The model under review builds one solid part; all positions refer to its coordinate system, in mm. A direction names the side the tool comes from. Coordinates: 2 decimals unless noted, no trailing zeros. Loops run counter-clockwise (first coordinate to the right, second up) from the corner with the lowest first, then second, coordinate; pieces in that order, holes last. Notation, with made-up numbers: M 26.25,17 L 42.25,17 A14 ccw 42.25,33 Z; hole C 71,86.5 d6. An arc over 180 degrees is marked long. Use one line per item in the form item = value.
```python
from build123d import *

# Parameters (mm, degrees)
F0_W     = 57
F0_H     = 44
F1_DEPTH = 167
F2_W     = 53
F2_H     = 40
F3_DEPTH = 165
F4_W     = 20
F4_H     = 15
F5_DEPTH = 84
F6_W     = 10
F6_H     = 80
F7_DEPTH = 2


with BuildPart() as f1:
    # F0 (on Top) → F1 (new body)
    with BuildSketch(Plane.XY):
        Rectangle(F0_W, F0_H)
    extrude(amount=F1_DEPTH)

    # F2 (on face) → F3 (cut)
    with BuildSketch(Plane.XY.offset(167)):
        Rectangle(F2_W, F2_H)
    extrude(amount=-F3_DEPTH, mode=Mode.SUBTRACT)

    # F4 (on face) → F5 (cut)
    with BuildSketch(Plane.YZ.offset(28.5)):
        with Locations((-12, 9.5)):
            Rectangle(F4_W, F4_H)
    extrude(amount=-F5_DEPTH, mode=Mode.SUBTRACT)

    # F6 (on face) → F7 (cut)
    with BuildSketch(Plane.XZ.offset(22)):
        Polygon((5, 49.017786), (-5, 49.017786), (0, 40.357532), align=None)
        with Locations((0, 89.017786)):
            Rectangle(F6_W, F6_H)
        Polygon((0, 137.67804), (-5, 129.017786), (5, 129.017786), align=None)
    extrude(amount=-F7_DEPTH, mode=Mode.SUBTRACT)


solid = f1.part
```
1. Add section B-B (z = 30). State the section outline as (x, y) points, then the cut area to 3 significant figures.
Response values:
outline = M -28.5,-22 L 28.5,-22 L 28.5,22 L -28.5,22 Z; hole M -26.5,-20 L 26.5,-20 L 26.5,20 L -26.5,20 Z
area = 388 mm^2
2. Wall thickness on line 1 along X through (y, z) = (11, 65); line 2 along Y through (x, z) = (-25.5, 136.5); line 3 along Z through (x, y) = (-18, -1): over which ranges is each line inside the solid? List them lowest first. Write a range as from..to.
Response values:
line_1 = -28.5..-26.5, 26.5..28.5
line_2 = -22..-20, 20..22
line_3 = 0..2
3. Add section A-A (x = -7). State the section outline as (y, z) points, then the cut area to 3 significant figures.
Response values:
outline = M -22,0 L 22,0 L 22,167 L 20,167 L 20,2 L -22,2 Z; M -22,17 L -20,17 L -20,167 L -22,167 Z
area = 718 mm^2
4. Add section D-D (x = 2). State the section outline as (y, z) points.
Response values:
outline = M -22,0 L 22,0 L 22,167 L 20,167 L 20,2 L -22,2 Z; M -22,17 L -20,17 L -20,43.82 L -22,43.82 Z; M -22,134.21 L -20,134.21 L -20,167 L -22,167 Z
5. The part is to be moulded in two halves that separate along Z. For faces 1 (the face through (6, -20, 93)), 2 (the face through (2.465, -21.014, 44.627)), 3 (the face through (0, 0, 0)), 4 (the face through (0.1, -20.2, 17)), say which applies: pulls with the +Z half, pulls with the -Z half, needs draft (parallel to the pull), parting line crosses it, or undercut.
Response values:
face_1 = needs draft
face_2 = undercut
face_3 = pulls with the -Z half
face_4 = undercut
6. Insertion check: P1, Ø1.5, axis at x = 3, y = 13.5, coming from the +Z side; P2, Ø12, axis at x = 14, y = 16, coming from the -Z side; P3, Ø1.6, axis at x = 27, z = 7.5, coming from the -Y side. Each pin has a flat end and moves straight along its axis. Give the tip position at first contact, or say it passes through.
Response values:
P1 = 2
P2 = 0
P3 = -2
7. Machinability: for faces 5 (the face through (2.535, -21.014, 133.287)), 6 (the face through (-26.5, 0, 86)), 7 (the face through (28.5, 0, 82)), which of the approach directions +Z, -Z, +X, -X, +Y, -Y give a long, thin tool a straight path to every point of the face, cutting with its end or side? Answer none if there is none.
Response values:
face_5 = -Y
face_6 = +Z
face_7 = +Z, -Z, +X, +Y, -Y
8. Add section C-C (y = -13.5). State the section outline as (x, z) points, then the cut area to 3 significant figures.
Response values:
outline = M -28.5,0 L 28.5,0 L 28.5,2 L -28.5,2 Z; M -28.5,17 L -26.5,17 L -26.5,167 L -28.5,167 Z; M 26.5,17 L 28.5,17 L 28.5,167 L 26.5,167 Z
area = 714 mm^2
